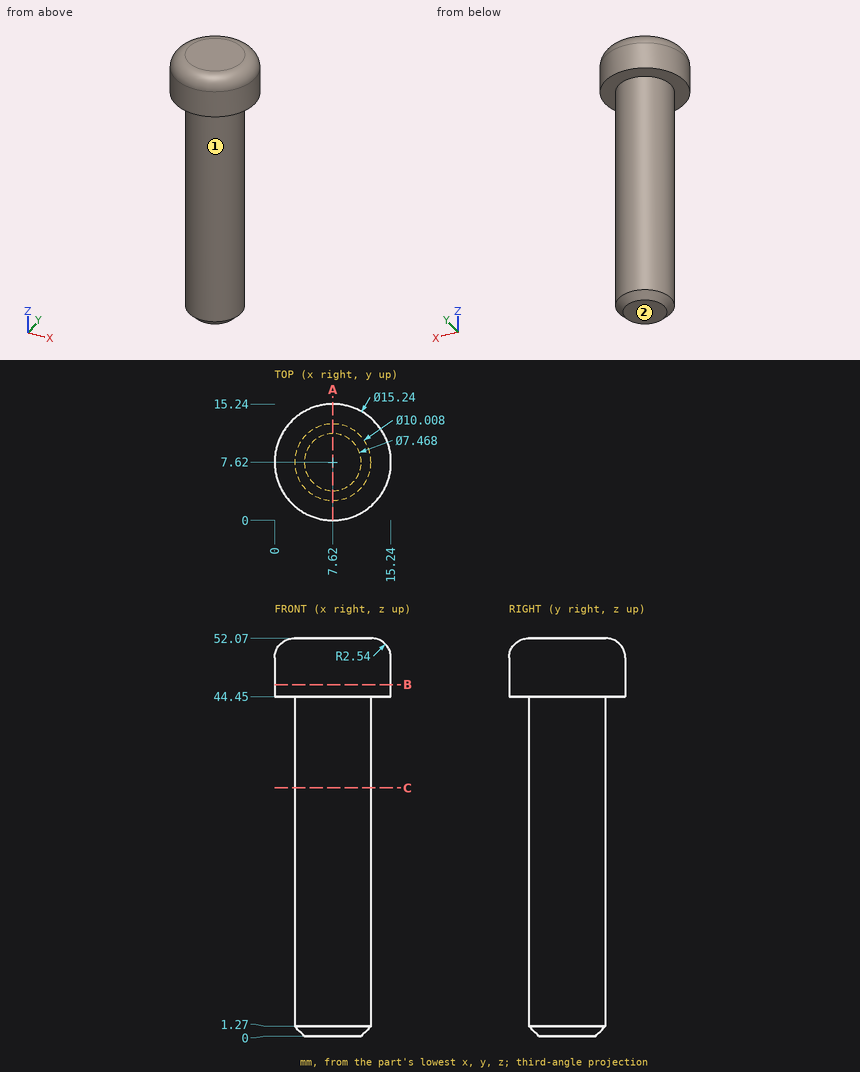
Could you check a few things on this drawing? It's one solid part, dimensions in mm from its lowest x, y, z. A direction names the side the tool comes from. Coordinates: 2 decimals unless noted, no trailing zeros. Order: outer loops, then holes, each group sorted by start corner. A loop starts at its lowest first (then second) coordinate and runs counter-clockwise, first axis right, second up. Notation, with made-up numbers: M -34,35 L 24,35 A10 cw 24,53 Z; hole C 3.5,-8.5 d3. An arc over 180 degrees is marked long. Use a Markdown table: item, result. Add a question column.
Q1. I'm going to push flat-ended pins straight in: pin 1 (6 mm diameter, centred on y = 8.5, z = 17.5, fed in from +X); pin 2 (8 mm diameter, centred on x = 3, z = 35, fed in from -Y) (1 decimal); pin 3 (6 mm diameter, centred on x = 2.5, y = 13, fed in from -Z). Where does each tip first touch, or does it pass through?
Q2. I want a section at A-A on x = 7.62. List the corners of the cut face in (y, z) for me.
Q3. Which directions (+Z, -Z, +X, -X, +Y, -Y) give clear straight access to the entire face, cutting with the end or side of a thin tool? Please do the marked faces 1 and 2.
Q4. I want a section at C-C on z = 32.5. List the corners of the cut face in (x, y) for me.
Q5. I want a section at B-B on z = 46. List the corners of the cut face in (x, y) for me.
Q6. If I drill on L1, parallel to X at y = 7.75, z = 35.5; L2, parallel to Z at x = 4, y = 9.75 (1 decimal); L3, parallel to Z at x = 3.75, y = 5.75 (1 decimal), over which ranges is the centre line in solid material (lowest first)?
Checked values:
| question | item | result |
|---|---|---|
| 1 | pin 1 | x = 12.62 |
| 1 | pin 2 | y = 2.7 |
| 1 | pin 3 | z = 0.69 |
| 2 | outline | M 0,44.45 L 2.62,44.45 L 2.62,1.27 L 3.89,0 L 11.35,0 L 12.62,1.27 L 12.62,44.45 L 15.24,44.45 L 15.24,49.53 A2.54 ccw 12.7,52.07 L 2.54,52.07 A2.54 ccw 0,49.53 Z |
| 3 | face 1 | -Z |
| 3 | face 2 | -Z, +X, -X, +Y, -Y |
| 4 | outline | C 7.62,7.62 d10.01 |
| 5 | outline | C 7.62,7.62 d15.24 |
| 6 | L1 | 2.62 to 12.62 |
| 6 | L2 | 0.5 to 52.1 |
| 6 | L3 | 0.6 to 52.1 |
